Study the drawing (mm; zero at the part's minimum x, y, z) and answer. Give positions to 0.01 mm unless a question says otherwise; leave off trailing zeros. Write each loop counter-clockwise with the first axis right and the second up, starting at its lowest first coordinate (ties: lowest second). Pieces come first, ordered by that corner, then holes.
1) Find section B-B (x = 25). Determine the outline of the cut face in (y, z).
2) Straight lines are drawn through the part: probe 1 along Y at (x, z) = (25, 1.55); probe 2 along Z at (x, y) = (21.5, 21); probe 3 along X at (y, z) = (13.5, 3). For each, find the intervals that lie inside material, in ascending order.
3) Find section C-C (z = 1.5). Determine the outline of the cut face in (x, y), plus the area to 3 significant figures.
4) Find section A-A (y = 11). Determine the outline of the cut face in (x, z).
5) Given pin 1 Ø1.2 at (x, z) = (10, 2.5) entering from -Y; pin 2 Ø4.5 at (y, z) = (7, 1.5) entering from -X; pin 3 Ø3 at (y, z) = (12, 2.5) entering from +X, each flat-ended and moving along its own axis, determine where each tip first touches the part or whether it passes through.
6) Find section D-D (x = 31). Determine the outline of the cut face in (y, z), plus the area to 3 significant figures.
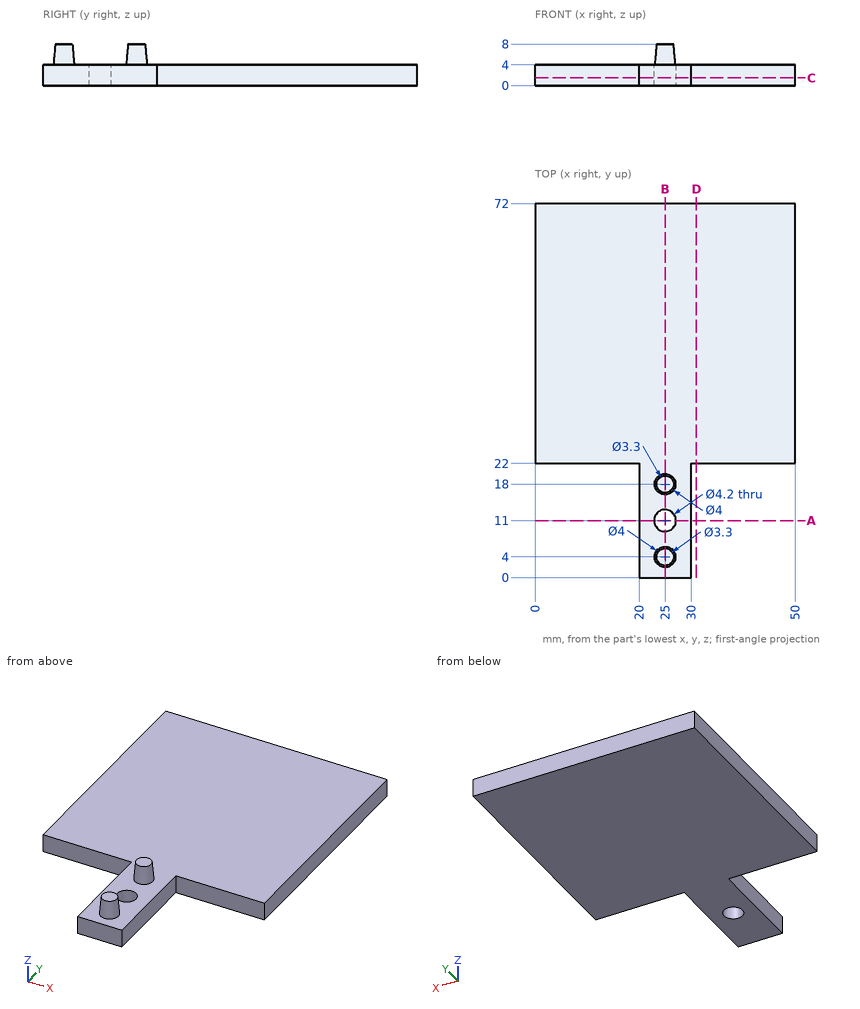
Results:
1. outline: (0, 0) - (8.9, 0) - (8.9, 4) - (6, 4) - (5.65, 8) - (2.35, 8) - (2, 4) - (0, 4) - close; (13.1, 0) - (72, 0) - (72, 4) - (20, 4) - (19.65, 8) - (16.35, 8) - (16, 4) - (13.1, 4) - close
2. probe 1: y = 0 to 8.9, 13.1 to 72
2. probe 2: z = 0 to 4
2. probe 3: x = 20 to 30
3. outline: (0, 22) - (20, 22) - (20, 0) - (30, 0) - (30, 22) - (50, 22) - (50, 72) - (0, 72) - close; hole circle Ø4.2 at (25, 11)
3. area: 2,710 mm2
4. outline: (20, 0) - (22.9, 0) - (22.9, 4) - (20, 4) - close; (27.1, 0) - (30, 0) - (30, 4) - (27.1, 4) - close
5. pin 1: stops at y = 22
5. pin 2: stops at x = 20
5. pin 3: stops at x = 30
6. outline: (22, 0) - (72, 0) - (72, 4) - (22, 4) - close
6. area: 200 mm2
